from build123d import *

# Parameters (mm, degrees)
SKETCH1_R           = 2.25
SKETCH1_W           = 6.15
SKETCH1_H           = 19.05
BOSS_EXTRUDE1_DEPTH = 6.35
SKETCH13_W          = 16
SKETCH13_H          = 5
CUT_EXTRUDE1_DEPTH  = 10
CHAMFER1_SIZE2      = 10
CHAMFER1_SIZE       = 8
FILLET1_R           = 1.5


with BuildPart() as part:
    # Sketch1 → Boss-Extrude1 (new, symmetric)
    with BuildSketch(Plane.XY):
        with BuildLine():
            Line((0, -5), (30, -5))
            Line((30, -5), (30, -25.05))
            Line((30, -25.05), (38.15, -25.05))
            Line((38.15, -25.05), (38.15, 5))
            Line((38.15, 5), (0, 5))
            ThreePointArc((0, 5), (-5, 0), (0, -5))
        make_face()
        Circle(SKETCH1_R, mode=Mode.SUBTRACT)
        with Locations((25, -0.066795827)):
            Circle(SKETCH1_R, mode=Mode.SUBTRACT)
        with Locations((34.075, -14.525)):
            Rectangle(SKETCH1_W, SKETCH1_H, mode=Mode.SUBTRACT)
    extrude(amount=BOSS_EXTRUDE1_DEPTH, both=True)

    # Sketch13 → Cut-Extrude1 (cut)
    with BuildSketch(Plane.XZ.offset(5)):
        with Locations((3, 0)):
            Rectangle(SKETCH13_W, SKETCH13_H)
    extrude(amount=-CUT_EXTRUDE1_DEPTH, mode=Mode.SUBTRACT)

    # Chamfer1
    chamfer1_edges = [part.edges().sort_by_distance(p)[0] for p in [
        (11, -5, 0),
    ]]
    chamfer1_side = [part.faces().sort_by_distance(p)[0] for p in [
        (11.16, -5, 0),
    ]]
    chamfer(chamfer1_edges, length=CHAMFER1_SIZE - 0.0001, length2=CHAMFER1_SIZE2 - 0.0001, reference=chamfer1_side[0])  # a hair under: the kernel refuses the full size

    # Fillet1
    fillet1_edges = [part.edges().sort_by_distance(p)[0] for p in [
        (38.15, 5, 0),
        (38.15, -25.05, 0),
        (30, -25.05, 0),
        (30, -5, 0),
    ]]
    fillet(fillet1_edges, radius=FILLET1_R)


solid = part.part
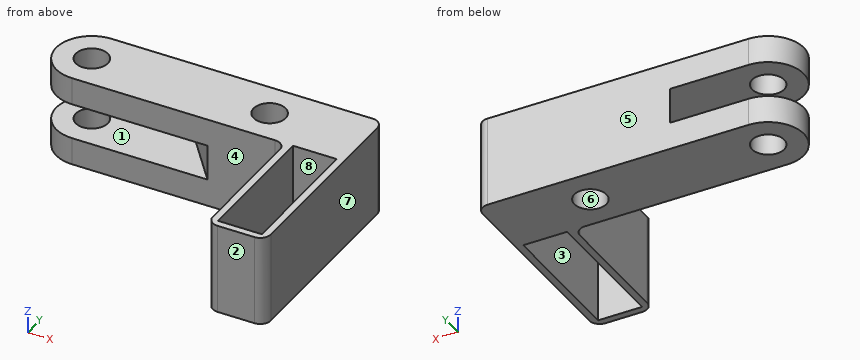
Can you work these out from the model? Positions are in its coordinate system, mm. Face numbers are marked on the shaded views. A direction names the side the tool comes from. Give positions to 0.01 mm unless a question says otherwise; leave off trailing zeros. Loops run counter-clockwise (first coordinate to the right, second up) from the corner with the lowest first, then second, coordinate; pieces in that order, holes last. Notation, with made-up numbers: (14, -24) -> (47, -24) arc R21 cw to (47, -13) -> close; hole circle Ø2 at (76.25, 0.5). An arc over 180 degrees is marked (long way). Use one line per item in the form item = value.
1) I need wall thicknesses on line 1 along Z through (x, y) = (-2, 3); line 2 along X through (y, z) = (1, -4.5); line 3 along Y through (x, z) = (0, 4.3). Which ranges of each line are inside material? Lowest first, please.
Answers:
line_1 = -6.35 to -2.5, 2.5 to 6.35
line_2 = -4.9 to -2.02, 2.02 to 23.02, 26.98 to 38.15
line_3 = -5 to -2.25, 2.25 to 5
2) For the marked faces 1, 2, 3 and 4, which set-ups out of +Z, -Z, +X, -X, +Y, -Y let a thin tool reach every point of the face, with its end or its side?
Answers:
face_1 = -X, -Y
face_2 = +Z, -Z, +X, -X, -Y
face_3 = +Z, -Z
face_4 = +Z, -Z, -X, -Y
3) We'd pull the mould along X, two halves only. Please class the marked faces 5, 6, 7 and 8: released by +X, released by -X, zero draft, split by the parting line, or undercut.
Answers:
face_5 = zero draft
face_6 = undercut
face_7 = released by +X
face_8 = undercut
4) Will these pins go through, and if not, where does the flat tip stop? pin 1 (2 mm diameter, centred on x = 31, z = 2.5, fed in from -Y); pin 2 (3 mm diameter, centred on x = 13, z = -4, fed in from -Y).
Answers:
pin_1 = -25.05
pin_2 = -5
5) If we section it at D-D (y = 1.5): Please give me the cut outline in (x, z), plus the area to 3 significant figures.
Answers:
outline = (-4.77, -6.35) -> (-1.68, -6.35) -> (-1.68, -2.5) -> (-4.77, -2.5) -> close; (-4.77, 2.5) -> (-1.68, 2.5) -> (-1.68, 6.35) -> (-4.77, 6.35) -> close; (1.68, -6.35) -> (23.39, -6.35) -> (23.39, 6.35) -> (1.68, 6.35) -> (1.68, 2.5) -> (13.8, 2.5) -> (13.8, -2.5) -> (1.68, -2.5) -> close; (26.61, -6.35) -> (38.15, -6.35) -> (38.15, 6.35) -> (26.61, 6.35) -> close
area = 385 mm²
6) If we section it at B-B (x = 10): Please give me the cut outline in (y, z).
Answers:
outline = (-5, -6.35) -> (5, -6.35) -> (5, -2.5) -> (-5, -2.5) -> close; (-5, 2.5) -> (5, 2.5) -> (5, 6.35) -> (-5, 6.35) -> close
7) If we section it at C-C (z = 1): Count the separate pieces of the cut face and the enclosed holes in it, plus the area to 3 significant figures.
Answers:
separate_pieces = 1
enclosed_holes = 2
area = 261 mm²
8) If we section it at A-A (y = -13): Please give me the cut outline in (x, z).
Answers:
outline = (30, -6.35) -> (31, -6.35) -> (31, 6.35) -> (30, 6.35) -> close; (37.15, -6.35) -> (38.15, -6.35) -> (38.15, 6.35) -> (37.15, 6.35) -> close
